Study the drawing (mm; zero at the part's minimum x, y, z) and answer. A direction names the side the tool comes from. Give positions to 0.01 mm unless a question says otherwise; leave off trailing zeros. Write each loop counter-clockwise with the first axis right and the second up, starting at its lowest first coordinate (ties: lowest second). Pieces come first, ordered by that corner, then holes. Notation, with made-up numbers: (29.5, 12) - (67.5, 12) arc R16 cw to (67.5, 38) - close; hole circle Ø4 at (-23, 31.5). An arc over 180 degrees is marked (long way). Answer as CSV lines item,"result".
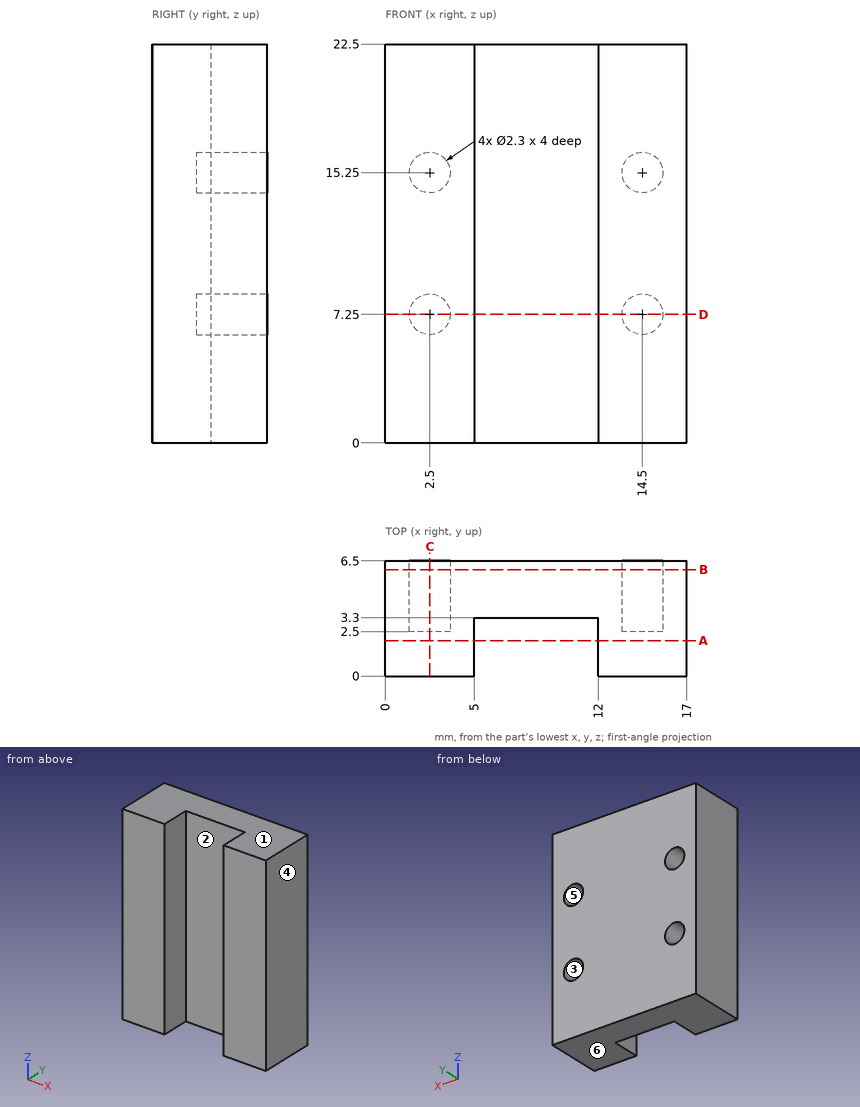
(1) A cutting plane is placed at D-D (z = 7.25). Write down the section's boundary in (x, y).
Worked out:
outline,"(0, 0) - (5, 0) - (5, 3.3) - (12, 3.3) - (12, 0) - (17, 0) - (17, 6.5) - (15.65, 6.5) - (15.65, 2.5) - (13.35, 2.5) - (13.35, 6.5) - (3.65, 6.5) - (3.65, 2.5) - (1.35, 2.5) - (1.35, 6.5) - (0, 6.5) - close"
(2) A cutting plane is placed at C-C (x = 2.5). Write down the section's boundary in (y, z), and give its area (3 significant figures).
Worked out:
outline,"(0, 0) - (6.5, 0) - (6.5, 6.1) - (2.5, 6.1) - (2.5, 8.4) - (6.5, 8.4) - (6.5, 14.1) - (2.5, 14.1) - (2.5, 16.4) - (6.5, 16.4) - (6.5, 22.5) - (0, 22.5) - close"
area,"128 mm^2"
(3) A cutting plane is placed at A-A (y = 2). Write down the section's boundary in (x, z).
Worked out:
outline,"(0, 0) - (5, 0) - (5, 22.5) - (0, 22.5) - close; (12, 0) - (17, 0) - (17, 22.5) - (12, 22.5) - close"
(4) This flat-tipped pin is pushed along its axis until it touches: P1, Ø1.1, axis at x = 15, z = 15, coming from the +Y side. Where does it stop, or does it pass through?
Worked out:
P1,"stops at y = 2.5"
(5) Find the intervals of material crossed by L1, parallel to Z at x = 2.5, y = 3.45; L2, parallel to X at y = 3.7, z = 7.25; L3, parallel to X at y = 2.25, z = 6.25, in increasing order.
Worked out:
L1,"z = 0 to 6.1, 8.4 to 14.1, 16.4 to 22.5"
L2,"x = 0 to 1.35, 3.65 to 13.35, 15.65 to 17"
L3,"x = 0 to 5, 12 to 17"
(6) The mould has two halves that part along Z. Classify the marked faces 4, 5 and 6: +Z half, -Z half, draft (parallel to the pull), parting line (faces both ways), or undercut.
Worked out:
face 4,"draft"
face 5,"undercut"
face 6,"-Z half"
(7) For the marked faces 1, 2 and 3, determine the directions among +Z, -Z, +X, -X, +Y, -Y from which every point of the face is accessible in a straight line to the end or side of a thin tool.
Worked out:
face 1,"+Z, +X, -X, +Y, -Y"
face 2,"+Z, -Z, -Y"
face 3,"+Y"
(8) A cutting plane is placed at B-B (y = 6). Write down the section's boundary in (x, z).
Worked out:
outline,"(0, 0) - (17, 0) - (17, 22.5) - (0, 22.5) - close; hole circle Ø2.3 at (2.5, 7.25); hole circle Ø2.3 at (2.5, 15.25); hole circle Ø2.3 at (14.5, 7.25); hole circle Ø2.3 at (14.5, 15.25)"
